from build123d import *

# Parameters (mm, degrees)
F0_R        = 1.625
F0_R_2      = 2.1
F1_DEPTH    = 9.5
F3_DEPTH    = 25
F4_T2_ANGLE = 184.9085480034
F4_T4_ANGLE = 184.9085480034
F4_T6_ANGLE = 184.9085480034
F4_T8_ANGLE = 184.9085480034


# Not quite as in the source:
# - a fillet or chamfer that OpenCascade refuses, or shapes differently, is made with other operations: its cross-section is extruded or revolved along the edge and cut away or added
# - a feature names something its author has since deleted; it is built from what else it names


with BuildPart() as f1:
    # F0 (on Front) → F1 (new body)
    with BuildSketch(Plane.XZ):
        with BuildLine():
            Line((-7.512280983, 15.2501027679), (-5.6857070658, 4.891087319))
            ThreePointArc((-5.6857070658, 4.891087319), (0, 7.5), (5.6857070658, 4.891087319))
            Line((5.6857070658, 4.891087319), (7.512280983, 15.2501027679))
            Line((7.512280983, 15.2501027679), (8.1508003801, 18.8713262163))
            Line((8.1508003801, 18.8713262163), (-1.2048732735, 20.5209839042))
            Line((-1.2048732735, 20.5209839042), (-1.8433926706, 16.8997604558))
            ThreePointArc((-1.8433926706, 16.8997604558), (-4.75, 16.3229133429), (-7.512280983, 15.2501027679))
        make_face()
        with Locations((-1.2020773276, 11.4370017967)):
            Circle(F0_R, mode=Mode.SUBTRACT)
        with BuildLine():
            ThreePointArc((-5.6857070658, 4.891087319), (-7.452634421, 0.8415700723), (-6.6332495807, -3.5))
            Line((-6.6332495807, -3.5), (6.6332495807, -3.5))
            ThreePointArc((6.6332495807, -3.5), (7.2800883187, -1.8028627436), (7.5, 0))
            ThreePointArc((7.5, 0), (7.0318135283, 2.6083708523), (5.6857070658, 4.891087319))
            ThreePointArc((5.6857070658, 4.891087319), (0, 7.5), (-5.6857070658, 4.891087319))
        make_face()
        Circle(F0_R_2, mode=Mode.SUBTRACT)
        with BuildLine():
            ThreePointArc((-6.6332495807, -3.5), (-5.9507591554, -4.5649168092), (-5.0990195136, -5.5))
            Line((-5.0990195136, -5.5), (0, -5.5))
            ThreePointArc((0, -5.5), (0.574906548, -5.4698704245), (1.1435142995, -5.379811804))
            Line((1.1435142995, -5.379811804), (6.1311080028, -4.3196660355))
            ThreePointArc((6.1311080028, -4.3196660355), (6.3953240131, -3.9178860075), (6.6332495807, -3.5))
            Line((6.6332495807, -3.5), (-6.6332495807, -3.5))
        make_face()
    extrude(amount=F1_DEPTH)

    # F2 (on face) → F3 (join)
    with BuildSketch(Plane(origin=(3.4729635533, 0, 19.6961550602), x_dir=(0.984807753, 0, -0.1736481777), z_dir=(0.1736481777, 0, 0.984807753))):
        with BuildLine():
            Line((4.75, -5.7297958971), (4.75, -3.7702041029))
            ThreePointArc((4.75, -3.7702041029), (3.4294678888, -1.3205321112), (0.9797958971, 0))
            Line((0.9797958971, 0), (-0.9797958971, 0))
            ThreePointArc((-0.9797958971, 0), (-3.4294678888, -1.3205321112), (-4.75, -3.7702041029))
            Line((-4.75, -3.7702041029), (-4.75, -5.7297958971))
            ThreePointArc((-4.75, -5.7297958971), (-3.4294678888, -8.1794678888), (-0.9797958971, -9.5))
            Line((-0.9797958971, -9.5), (0.9797958971, -9.5))
            ThreePointArc((0.9797958971, -9.5), (3.4294678888, -8.1794678888), (4.75, -5.7297958971))
        make_face()
    extrude(amount=F3_DEPTH)

    # F4: fillet of radius 2 on 4 edges, made by hand

    # F4_s1 → F4_t2 (revolve, cut)
    with BuildSketch(Plane(origin=(2.3303405276, -2.5782182234, -0.4109019093), x_dir=(-0.7418696826, -0.6705440881, 0), z_dir=(-0.6659057216, 0.7367379343, 0.1174171453))):
        with BuildLine():
            ThreePointArc((2.4557468395, 43.6793554426), (1.6921353384, 45.0072275442), (0.2132331001, 45.4062200412))
            Line((0.2132331001, 45.4062200412), (0.187450643, 45.6046889581))
            ThreePointArc((0.187450643, 45.6046889581), (1.1796484238, 45.7331788115), (2.1717946748, 45.8620653318))
            Line((2.1717946748, 45.8620653318), (2.3960460488, 45.6893788719))
            ThreePointArc((2.3960460488, 45.6893788719), (2.5249325691, 44.6972326209), (2.6542157564, 43.7051378996))
            Line((2.6542157564, 43.7051378996), (2.4557468395, 43.6793554426))
        make_face()
    revolve(axis=Axis((7.814167995, -4.75, 44.3163488855), (0.1736481777, 0, 0.984807753)), revolution_arc=F4_T2_ANGLE, mode=Mode.SUBTRACT)

    # F4_s3 → F4_t4 (revolve, cut)
    with BuildSketch(Plane(origin=(-2.3303405276, -2.1717817766, 0.4109019093), x_dir=(0.6817807283, -0.731556586, 0), z_dir=(-0.7255452297, -0.6761783908, 0.1279331997))):
        with BuildLine():
            ThreePointArc((13.3818366305, 41.7080845524), (12.9673157833, 43.1827096947), (11.6314878435, 43.9323166305))
            Line((11.6314878435, 43.9323166305), (11.655182008, 44.1310456738))
            ThreePointArc((11.655182008, 44.1310456738), (12.6485812749, 44.0122013421), (13.6420278977, 43.8937541973))
            Line((13.6420278977, 43.8937541973), (13.8170627765, 43.6713309895))
            ThreePointArc((13.8170627765, 43.6713309895), (13.6986156317, 42.6778843667), (13.5805656738, 41.6843903878))
            Line((13.5805656738, 41.6843903878), (13.3818366305, 41.7080845524))
        make_face()
    revolve(axis=Axis((7.814167995, -4.75, 44.3163488855), (0.1736481777, 0, 0.984807753)), revolution_arc=F4_T4_ANGLE, mode=Mode.SUBTRACT)

    # F4_s5 → F4_t6 (revolve, cut)
    with BuildSketch(Plane(origin=(2.3303405276, -2.5782182234, -0.4109019093), x_dir=(0.7418696826, 0.6705440881, 0), z_dir=(0.6659057216, -0.7367379343, -0.1174171453))):
        with BuildLine():
            ThreePointArc((5.4373559827, 44.6721702336), (6.7652280844, 43.9085587325), (7.1642205814, 42.4296564942))
            Line((7.1642205814, 42.4296564942), (7.3626894983, 42.4038740371))
            ThreePointArc((7.3626894983, 42.4038740371), (7.4911793516, 43.3960718179), (7.6200658719, 44.3882180689))
            Line((7.6200658719, 44.3882180689), (7.4473794121, 44.6124694429))
            ThreePointArc((7.4473794121, 44.6124694429), (6.455233161, 44.7413559632), (5.4631384397, 44.8706391505))
            Line((5.4631384397, 44.8706391505), (5.4373559827, 44.6721702336))
        make_face()
    revolve(axis=Axis((7.814167995, -4.75, 44.3163488855), (0.1736481777, 0, 0.984807753)), revolution_arc=F4_T6_ANGLE, mode=Mode.SUBTRACT)

    # F4_s7 → F4_t8 (revolve, cut)
    with BuildSketch(Plane(origin=(-2.3303405276, -2.1717817766, 0.4109019093), x_dir=(-0.6817807283, 0.731556586, 0), z_dir=(0.7255452297, 0.6761783908, -0.1279331997))):
        with BuildLine():
            ThreePointArc((-5.9734927288, 44.6069108674), (-4.4988675865, 44.1923900202), (-3.7492606507, 42.8565620804))
            Line((-3.7492606507, 42.8565620804), (-3.5505316074, 42.880256245))
            ThreePointArc((-3.5505316074, 42.880256245), (-3.669375939, 43.8736555118), (-3.7878230838, 44.8671021347))
            Line((-3.7878230838, 44.8671021347), (-4.0102462916, 45.0421370134))
            ThreePointArc((-4.0102462916, 45.0421370134), (-5.0036929145, 44.9236898686), (-5.9971868933, 44.8056399107))
            Line((-5.9971868933, 44.8056399107), (-5.9734927288, 44.6069108674))
        make_face()
    revolve(axis=Axis((7.814167995, -4.75, 44.3163488855), (0.1736481777, 0, 0.984807753)), revolution_arc=F4_T8_ANGLE, mode=Mode.SUBTRACT)


solid = f1.part
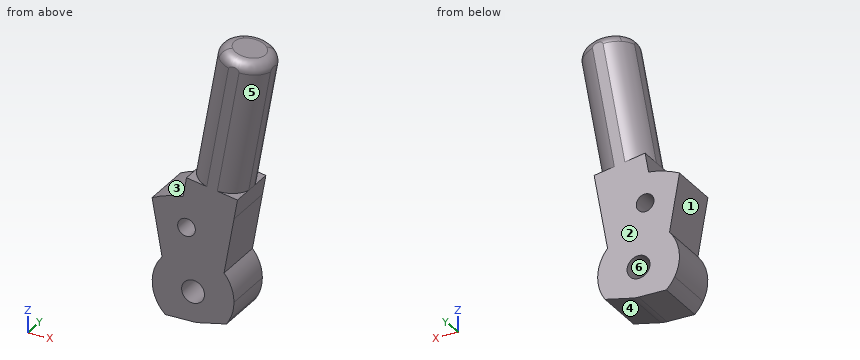
For this review, take the finished solid that the model builds, in its own axes (mm). Face numbers are marked on the shaded views. A direction names the side the tool comes from. Round coordinates to 2 decimals unless told otherwise and drop trailing zeros. Loops run counter-clockwise (first coordinate to the right, second up) from the corner with the lowest first, then second, coordinate; pieces in that order, holes last. Notation, with made-up numbers: (4.25, 42.5) - (55.25, 42.5) arc R17 ccw to (55.25, 58.5) - close; hole circle Ø3 at (29.25, -36). An arc over 180 degrees is marked (long way). Put each result on its own line as item: value. Start each with the question number.
1. For probe 1 along Z at (x, y) = (-1, -2.25); probe 2 along X at (y, z) = (-7, 5.5); probe 3 along Z at (x, y) = (-5.5, -4.5), list the stretches that pass through material, from the lowest coordinate up. Write a range as [from, to].
2. Consider section B-B on y = -5.25. State how many separate pieces and enclosed holes the cut face has, plus the area to 3 significant figures.
3. Consider section A-A on z = 1.5. State the section outline as (x, y) points, plus the area to 3 significant figures.
4. Mouldability with a two-part tool opening along Z and no side actions: class the marked faces 3, 4, 5 and 6 as +Z half, -Z half, draft (parallel to the pull), parting line (faces both ways), or undercut.
5. Consider section C-C on z = 7. State the section outline as (x, y) points, plus the area to 3 significant figures.
6. Insertion check: P1, Ø10, axis at x = -1.5, z = 36.5, coming from the +Y side; P2, Ø1.9, axis at x = -1.2, z = 11.44, coming from the +Y side; P3, Ø1, axis at y = -5, z = 36, coming from the -X side; P4, Ø5, axis at y = -5, z = 26.5, coming from the +X side. Each pin has a flat end and moves straight along its axis. Give the tip position at first contact, or say it passes through.
7. For the marked faces 1 and 2, list the 3-axis set-ups (+Z, -Z, +X, -X, +Y, -Y) from which the entire face can be reached by the end or side of a thin tool; tool diameter is ignored.
Result sheet:
1. probe 1: [-5.5, -1.85], [1.85, 9.82], [13.05, 20.48]
1. probe 2: [-5.79, 5.79]
1. probe 3: [-5.1, 16.09]
2. separate pieces: 1
2. enclosed holes: 2
2. area: 538 mm^2
3. outline: (-7.35, -9.5) - (-1.47, -9.5) - (-1.47, 0) - (-7.35, 0) - close; (1.47, -9.5) - (7.35, -9.5) - (7.35, 0) - (1.47, 0) - close
3. area: 112 mm^2
4. face 3: +Z half
4. face 4: -Z half
4. face 5: undercut
4. face 6: undercut
5. outline: (-6.06, -9.5) - (6.06, -9.5) - (6.06, 0) - (-6.06, 0) - close
5. area: 115 mm^2
6. P1: y = -0.8
6. P2: through
6. P3: x = 1.44
6. P4: x = 9.94
7. face 1: -X, +Y, -Y
7. face 2: +Z, -Z, +X, -X, +Y
